from build123d import *

# Parameters (mm, degrees)
SKETCH1_W               = 80
SKETCH1_H               = 100
SKETCH1_W_2             = 60
SKETCH1_H_2             = 80
EXTRUDE_THIN1_DEPTH     = 10
BOSS_EXTRUDE1_DEPTH     = 10
CUT_EXTRUDE1_REACH      = 200.286
SKETCH3_R               = 5
CUT_EXTRUDE2_DEPTH      = 191.061213228
CUT_EXTRUDE2_DEPTH_BACK = 191.061213228
SKETCH4_R               = 2.5


with BuildPart() as part:
    # Sketch1 → Extrude-Thin1 (new, symmetric)
    with BuildSketch(Plane.XY):
        with Locations((50, -140)):
            Rectangle(SKETCH1_W, SKETCH1_H)
        with Locations((50, -140)):
            Rectangle(SKETCH1_W_2, SKETCH1_H_2, mode=Mode.SUBTRACT)
    extrude(amount=EXTRUDE_THIN1_DEPTH, both=True)

    # Sketch2 → Boss-Extrude1 (add, symmetric)
    with BuildSketch(Plane.XY):
        Polygon((27.071067812, -92.928932188), (-47.175144213, -18.682720164), (-61.317279836, -32.824855787), (12.928932188, -107.071067812), align=None)
    boss_extrude1 = extrude(amount=BOSS_EXTRUDE1_DEPTH, both=True)

    # Sketch3 → Cut-Extrude1 (cut, up to next)
    with BuildSketch(Plane(origin=(-47.071067812, -47.071067812, 0), x_dir=(0, 0, 1), z_dir=(-0.7071067811865477, -0.7071067811865475, 0)), mode=Mode.PRIVATE) as cut_extrude1_sk1:
        with Locations(Location((0, 8.485281374, 0), (0, 0, 270))):
            Circle(SKETCH3_R)
    cut_extrude1_tool1 = extrude(cut_extrude1_sk1.sketch, amount=-CUT_EXTRUDE1_REACH, mode=Mode.PRIVATE) & part.part
    cut_extrude1 = cut_extrude1_tool1.solids().sort_by_distance((-53.071068, -41.071068, 0))[0]
    add(cut_extrude1, mode=Mode.SUBTRACT)

    # Mirror1: Boss-Extrude1, Cut-Extrude1 across plane
    add(boss_extrude1.mirror(Plane(origin=(50, 0, 0), x_dir=(0, 0, 1), z_dir=(1, 0, 0))))
    add(cut_extrude1.mirror(Plane(origin=(50, 0, 0), x_dir=(0, 0, 1), z_dir=(1, 0, 0))), mode=Mode.SUBTRACT)

    # Sketch4 → Cut-Extrude2 (cut, two sides: drawn at the far end of the back side and taken through both)
    with BuildSketch(Plane(origin=(0, -90, 0), x_dir=(1, 0, 0), z_dir=(0, 1, 0)).offset(-CUT_EXTRUDE2_DEPTH_BACK)):
        with Locations(Location((50, 0, 0), (0, 0, 270))):
            Circle(SKETCH4_R)
    extrude(amount=CUT_EXTRUDE2_DEPTH + CUT_EXTRUDE2_DEPTH_BACK, mode=Mode.SUBTRACT)


solid = part.part
Part model, mm, in its own coordinate system. A direction names the side the tool comes from. Give positions to 0.01 mm unless a question says otherwise; leave off trailing zeros. Loops run counter-clockwise (first coordinate to the right, second up) from the corner with the lowest first, then second, coordinate; pieces in that order, holes last. Notation, with made-up numbers: M 14,64.25 L 35,64.25 A21 ccw 35,77.25 Z; hole C -15.75,80.25 d4. An arc over 180 degrees is marked long. Put each result on its own line as item: value. Start each with the question number.
1) Saw through at B-B (y = -81). List the corners of the cut face in (x, z), then the cut area to 3 significant figures.
2) Saw through at C-C (z = 0). State how many separate pieces and enclosed holes the cut face has, then the cut area to 3 significant figures.
3) Flat gauge pins, fed straight in: pin 1 (3 mm diameter, centred on x = 50, z = 0, fed in from -Y); pin 2 (10 mm diameter, centred on y = -127, z = 3.5, fed in from -X); pin 3 (8 mm diameter, centred on x = 13, z = -1, fed in from +Y); pin 4 (6 mm diameter, centred on y = -136, z = -1, fed in from +X). Where does each tip first touch, or does it go through?
4) Pull direction Z, two halves, no side cores. Call faces 6 (the flat face through (49, -98, 10)), 7 (the flat face through (51, -98, -10)), 8 (the flat face through (80, -141, 0)), 9 (the cylindrical face through (47.56, -95.07, -0.54)): +Z half, -Z half, draft (parallel to the pull), parting line (faces both ways), or undercut.
5) Saw through at A-A (x = 50). List the corners of the cut face in (y, z), then the cut area to 3 significant figures.
6) 3-axis set-ups, long thin cutter, end or side, ignore diameter. For faces 1 (the flat face through (49, -190, 5)), 2 (the flat face through (10, -148, 0)), 3 (the flat face through (50, -100, 5)), 4 (the flat face through (-11.02, -54.84, 0.14)), 5 (the flat face through (90, -148, 0)): which of +Z, -Z, +X, -X, +Y, -Y reach the whole face in a straight line?
7) Probe probe 1 along X at (y, z) = (-166.5, -8.25); probe 2 along Y at (x, z) = (44, -4); probe 3 along Z at (x, y) = (50, -184). List the from-to ranges inside material, lowest first.
Numbers:
1. outline: M -13.14,-10 L 15.14,-10 L 15.14,10 L -13.14,10 Z; M 84.86,-10 L 113.14,-10 L 113.14,10 L 84.86,10 Z
1. area: 1,130 mm^2
2. separate pieces: 4
2. enclosed holes: 0
2. area: 6,530 mm^2
3. pin 1: through
3. pin 2: x = 10
3. pin 3: y = -74.86
3. pin 4: x = 90
4. face 6: +Z half
4. face 7: -Z half
4. face 8: draft
4. face 9: undercut
5. outline: M -190,-10 L -180,-10 L -180,-2.5 L -190,-2.5 Z; M -190,2.5 L -180,2.5 L -180,10 L -190,10 Z; M -100,-10 L -90,-10 L -90,-2.5 L -100,-2.5 Z; M -100,2.5 L -90,2.5 L -90,10 L -100,10 Z
5. area: 300 mm^2
6. face 1: +Z, -Z, +X, -X, -Y
6. face 2: +Z, -Z, -X, -Y
6. face 3: +Z, -Z
6. face 4: +Z, -Z, +Y
6. face 5: +Z, -Z, +X, -Y
7. probe 1: 10 to 20, 80 to 90
7. probe 2: -190 to -180, -100 to -90
7. probe 3: -10 to -2.5, 2.5 to 10
